The model under review builds one solid part; all positions refer to its coordinate system, in mm. Face numbers are marked on the shaded views. A direction names the side the tool comes from. Round coordinates to 2 decimals unless told otherwise and drop trailing zeros. Order: outer loops, then holes, each group sorted by start corner. A loop starts at its lowest first (then second) coordinate and runs counter-clockwise, first axis right, second up.
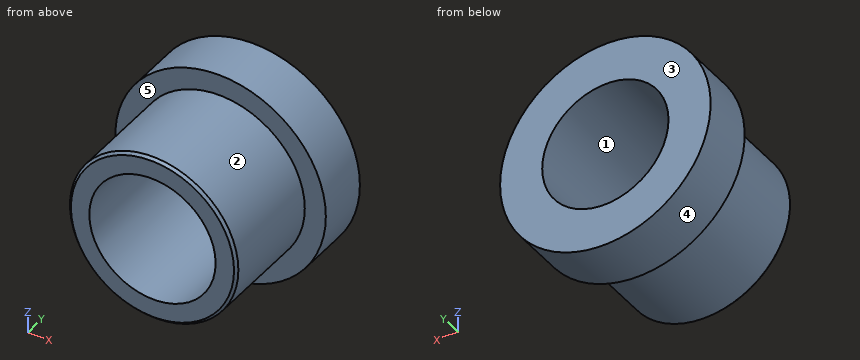
```python
from build123d import *

# Parameters (mm, degrees)
F0_R     = 8
F0_R_2   = 6
F1_DEPTH = 15
F0_R_3   = 10
F2_DEPTH = 5
F3_SIZE  = 0.25


with BuildPart() as f1:
    # F0 (on Front) → F1 (new body)
    with BuildSketch(Plane.XZ):
        Circle(F0_R)
        Circle(F0_R_2, mode=Mode.SUBTRACT)
    extrude(amount=F1_DEPTH)

    # F0 (on Front) → F2 (join)
    with BuildSketch(Plane.XZ):
        Circle(F0_R_3)
        Circle(F0_R, mode=Mode.SUBTRACT)
    extrude(amount=F2_DEPTH)

    # F3
    f3_edges = [f1.edges().sort_by_distance(p)[0] for p in [
        (-8, -15, 0),
    ]]
    chamfer(f3_edges, length=F3_SIZE)


solid = f1.part
```
(1) Consider section A-A (z = 0). Write out the cut boundary in (x, y), and give its area (3 significant figures).
Data:
outline: (-10, -5) - (-8, -5) - (-8, -14.75) - (-7.75, -15) - (-6, -15) - (-6, 0) - (-10, 0) - close; (6, -15) - (7.75, -15) - (8, -14.75) - (8, -5) - (10, -5) - (10, 0) - (6, 0) - close
area: 79.9 mm2
(2) To check wall thickness, follow probe 1 along Z at (x, y) = (0, -11.5); probe 2 along Y at (x, z) = (5, 7); probe 3 along Z at (x, y) = (0, -4.25). State the ranges of each line that lie inside material, in increasing order.
Data:
probe 1: z = -8 to -6, 6 to 8
probe 2: y = -5 to 0
probe 3: z = -10 to -6, 6 to 10
(3) Insertion check: pin 1 (5 mm diameter, centred on y = -10.5, z = 3.5, fed in from -X); pin 2 (11 mm diameter, centred on x = 0, z = 0, fed in from +Y); pin 3 (1 mm diameter, centred on x = 7, y = -7.5, fed in from -Z); pin 4 (1 mm diameter, centred on x = -1, y = -7, fed in from +Z). Each pin has a flat end and moves straight along its axis. Give the tip position at first contact, or say it passes through.
Data:
pin 1: stops at x = -7.94
pin 2: passes through
pin 3: stops at z = -4.66
pin 4: stops at z = 7.98
(4) For the marked faces 4 and 5, list the 3-axis set-ups (+Z, -Z, +X, -X, +Y, -Y) from which the entire face can be reached by the end or side of a thin tool; tool diameter is ignored.
Data:
face 4: +Y, -Y
face 5: -Y
(5) Consider section C-C (y = -14). Write out the cut boundary in (x, z).
Data:
outline: circle Ø16 at (0, 0); hole circle Ø12 at (0, 0)
(6) Consider section D-D (y = -4). Write out the cut boundary in (x, z), and give its area (3 significant figures).
Data:
outline: circle Ø20 at (0, 0); hole circle Ø12 at (0, 0)
area: 201 mm2
(7) Draft analysis for pull direction Z (two halves, no side actions). For the marked faces 1, 2 and 3, state which applies: pulls with the +Z half, pulls with the -Z half, needs draft (parallel to the pull), parting line crosses it, or undercut.
Data:
face 1: undercut
face 2: parting line crosses it
face 3: needs draft
(8) Consider section B-B (x = 0). Write out the cut boundary in (y, z).
Data:
outline: (-15, -7.75) - (-14.75, -8) - (-5, -8) - (-5, -10) - (0, -10) - (0, -6) - (-15, -6) - close; (-15, 6) - (0, 6) - (0, 10) - (-5, 10) - (-5, 8) - (-14.75, 8) - (-15, 7.75) - close
